Verification items for the finished model (mm, model axes). Coordinates: 2 decimals unless noted, no trailing zeros. Order: outer loops, then holes, each group sorted by start corner. A loop starts at its lowest first (then second) coordinate and runs counter-clockwise, first axis right, second up.
Q1. Cross-section at B-B, the plane x = -19.05. Record the boundary of the cut face in (y, z), and give its area (3 significant figures).
Q2. Cross-section at C-C, the plane z = -2. Record the boundary of the cut face in (x, y).
Q3. Thickness scan on line 1 (X direction, y = -6.35, z = -5.55); line 2 (Y direction, x = 19.05, z = -4.7); line 3 (X direction, y = -8.5, z = -0.75). Record the ranges inside material, lowest first.
Q4. Depth check by flat-ended pin: P1, Ø4, axis at x = 19.05, y = -6.35, coming from the -Z side; P2, Ø11, axis at x = -19.05, y = -6.35, coming from the +Z side. Enter the tip coordinate at first touch or a pass-through.
Q5. Draft check along Y on faces 1 (the flat face through (-1, -12.7, -3)), 2 (the conical face through (19.511, -2.839, -3.684)), 3 (the flat face through (-38.1, 0, -3)), 4 (the flat face through (-1, 12.7, -3)). Enter one of: pulls with the +Y half, pulls with the -Y half, needs draft (parallel to the pull), parting line crosses it, or undercut.
Q6. Cross-section at A-A, the plane y = -6.35. Record the boundary of the cut face in (x, z).
from build123d import *

# Parameters (mm, degrees)
F0_W           = 76.2
F0_H           = 25.4
F0_R           = 3.571875
F1_DEPTH       = 6.35
F2_D           = 6.7564
F2_DEPTH       = 19.05
F2_CSINK_D     = 13.4874
F2_CSINK_ANGLE = 82
F2_TIP         = 2.0298273432


with BuildPart() as f1:
    # F0 (on Top) → F1 (new body)
    with BuildSketch(Plane.XY):
        Rectangle(F0_W, F0_H)
        with Locations((-19.05, -6.35)):
            Circle(F0_R, mode=Mode.SUBTRACT)
        with Locations((19.05, -6.35)):
            Circle(F0_R, mode=Mode.SUBTRACT)
        with Locations((19.05, -6.35)):
            Circle(F0_R)
        with Locations((-19.05, -6.35)):
            Circle(F0_R)
    extrude(amount=-F1_DEPTH)

    # F2
    with Locations(Plane.XY):
        with Locations((-19.05, -6.35), (19.05, -6.35)):
            CounterSinkHole(F2_D / 2, F2_CSINK_D / 2, depth=F2_DEPTH, counter_sink_angle=F2_CSINK_ANGLE)
            with Locations((0, 0, -(F2_DEPTH + F2_TIP / 2))):  # 118° drill point
                Cone(0, F2_D / 2, F2_TIP, mode=Mode.SUBTRACT)


solid = f1.part
Check values:
1. outline: (-12.7, -6.35) - (-9.73, -6.35) - (-9.73, -3.87) - (-12.7, -0.45) - close; (-2.97, -6.35) - (12.7, -6.35) - (12.7, 0) - (0.39, 0) - (-2.97, -3.87) - close
1. area: 105 mm2
2. outline: (-38.1, -12.7) - (38.1, -12.7) - (38.1, 12.7) - (-38.1, 12.7) - close; hole circle Ø10.01 at (-19.05, -6.35); hole circle Ø10.01 at (19.05, -6.35)
3. line 1: x = -38.1 to -22.43, -15.67 to 15.67, 22.43 to 38.1
3. line 2: y = -12.7 to -9.73, -2.97 to 12.7
3. line 3: x = -38.1 to -24.75, -13.35 to 13.35, 24.75 to 38.1
4. P1: passes through
4. P2: stops at z = -1.43
5. face 1: pulls with the -Y half
5. face 2: undercut
5. face 3: needs draft
5. face 4: pulls with the +Y half
6. outline: (-38.1, -6.35) - (-22.43, -6.35) - (-22.43, -3.87) - (-25.79, 0) - (-38.1, 0) - close; (-15.67, -6.35) - (15.67, -6.35) - (15.67, -3.87) - (12.31, 0) - (-12.31, 0) - (-15.67, -3.87) - close; (22.43, -6.35) - (38.1, -6.35) - (38.1, 0) - (25.79, 0) - (22.43, -3.87) - close
